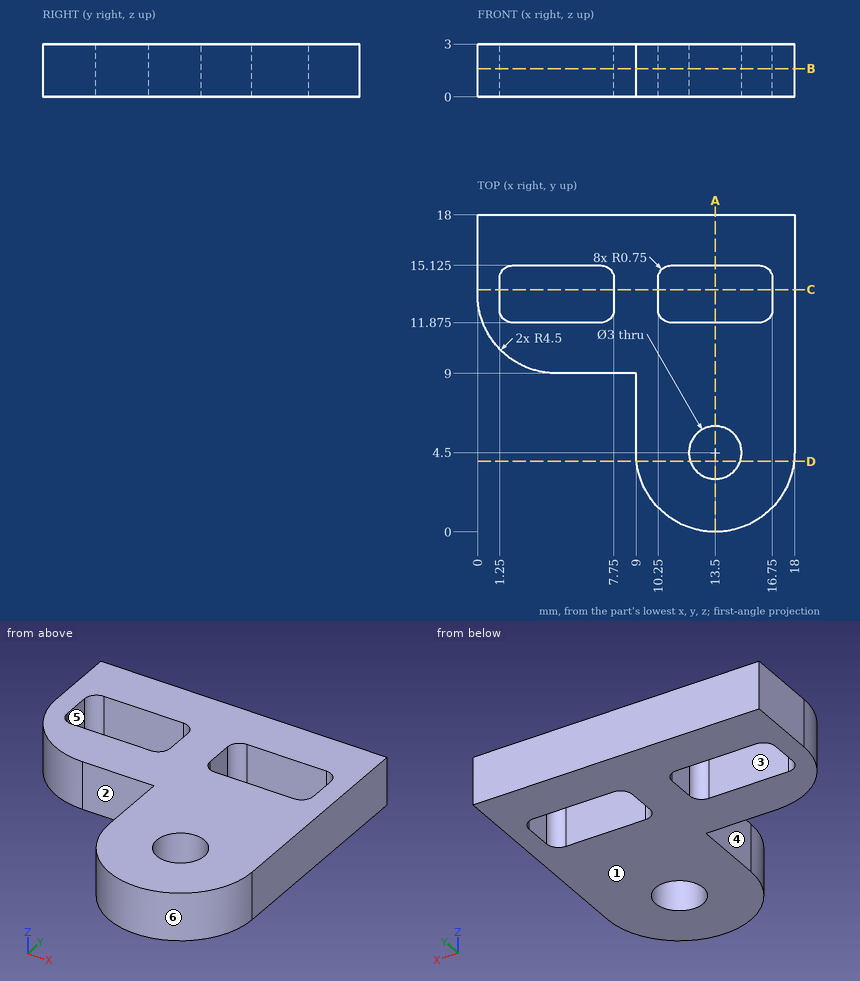
Part print with two shaded views. Sizes in mm from the minimum x, y, z corner. A direction names the side the tool comes from. Coordinates: 2 decimals unless noted, no trailing zeros. Loops run counter-clockwise (first coordinate to the right, second up) from the corner with the lowest first, then second, coordinate; pieces in that order, holes last. Notation, with made-up numbers: (32.25, 85) -> (90.25, 85) arc R28 cw to (90.25, 114) -> close; hole circle Ø1 at (40.5, 67). An arc over 180 degrees is marked (long way). Answer as a JSON object with one key per item and string values.
Q1. Cut at A-A (x = 13.5). List the corners of the cut face in (y, z) (3 decimals).
Report:
{"outline": "(0, 0) -> (3, 0) -> (3, 3) -> (0, 3) -> close; (6, 0) -> (11.875, 0) -> (11.875, 3) -> (6, 3) -> close; (15.125, 0) -> (18, 0) -> (18, 3) -> (15.125, 3) -> close"}
Q2. Cut at C-C (y = 13.75). List the corners of the cut face in (x, z), and give its area (3 significant figures).
Report:
{"outline": "(0, 0) -> (1.25, 0) -> (1.25, 3) -> (0, 3) -> close; (7.75, 0) -> (10.25, 0) -> (10.25, 3) -> (7.75, 3) -> close; (16.75, 0) -> (18, 0) -> (18, 3) -> (16.75, 3) -> close", "area": "15.0 mm2"}
Q3. Cut at B-B (z = 1.6). List the corners of the cut face in (x, y) (3 decimals).
Report:
{"outline": "(0, 13.5) arc R4.5 ccw to (4.5, 9) -> (9, 9) -> (9, 4.5) arc R4.5 ccw to (18, 4.5) -> (18, 18) -> (0, 18) -> close; hole (1.25, 12.625) arc R0.75 ccw to (2, 11.875) -> (7, 11.875) arc R0.75 ccw to (7.75, 12.625) -> (7.75, 14.375) arc R0.75 ccw to (7, 15.125) -> (2, 15.125) arc R0.75 ccw to (1.25, 14.375) -> close; hole (10.25, 12.625) arc R0.75 ccw to (11, 11.875) -> (16, 11.875) arc R0.75 ccw to (16.75, 12.625) -> (16.75, 14.375) arc R0.75 ccw to (16, 15.125) -> (11, 15.125) arc R0.75 ccw to (10.25, 14.375) -> close; hole circle Ø3 at (13.5, 4.5)"}
Q4. Cut at D-D (y = 4). List the corners of the cut face in (x, z), and give its area (3 significant figures).
Report:
{"outline": "(9.03, 0) -> (12.09, 0) -> (12.09, 3) -> (9.03, 3) -> close; (14.91, 0) -> (17.97, 0) -> (17.97, 3) -> (14.91, 3) -> close", "area": "18.3 mm2"}
Q5. 3-axis set-ups, long thin cutter, end or side, ignore diameter. For the marked faces 1, 2 and 3: which of +Z, -Z, +X, -X, +Y, -Y reach the whole face in a straight line?
Report:
{"face 1": "-Z, +X, -X, +Y, -Y", "face 2": "+Z, -Z, -X, -Y", "face 3": "+Z, -Z"}
Q6. Pull direction Y, two halves, no side cores. Call the marked faces 4, 5 and 6: released by +Y, released by -Y, zero draft, split by the parting line, or undercut.
Report:
{"face 4": "zero draft", "face 5": "undercut", "face 6": "released by -Y"}
Q7. Probe probe 1 along Y at (x, z) = (13.5, 1.85) (3 decimals); probe 2 along X at (y, z) = (14.25, 2.6); probe 3 along X at (y, z) = (4.5, 1.55). List the from-to ranges inside material, lowest first.
Report:
{"probe 1": "y = 0 to 3, 6 to 11.875, 15.125 to 18", "probe 2": "x = 0 to 1.25, 7.75 to 10.25, 16.75 to 18", "probe 3": "x = 9 to 12, 15 to 18"}
Q8. Flat gauge pins, fed straight in: P1, Ø1, axis at x = 16, z = 2, coming from the -Y side; P2, Ø1.5, axis at x = 7, z = 1, coming from the -Y side; P3, Ø1.5, axis at y = 6.5, z = 1, coming from the -X side. Where does each tip first touch, or does it go through?
Report:
{"P1": "stops at y = 0.47", "P2": "stops at y = 9", "P3": "stops at x = 9"}
